Input: part model. Units: mm. Frame: model coordinates. Face numbers are marked on the shaded views. Coordinates: 2 decimals unless noted, no trailing zeros. Order: outer loops, then holes, each group sorted by start corner. A loop starts at its lowest first (then second) coordinate and runs counter-clockwise, first axis right, second up. Notation, with made-up numbers: (31.5, 41.25) -> (61.5, 41.25) arc R16 ccw to (61.5, 54.25) -> close; hole circle Ø4 at (0.25, 71.5). An arc over 180 degrees is marked (long way). Use one line per item in the form item = value. Start each with the question number.
1) Ray query, line 1 along X through (y, z) = (3, 0.5); line 2 along Z through (x, y) = (32.5, 0); line 3 along Y through (x, z) = (9, 0.25). Return the intervals inside material, ascending.
2) Pin query (flat end, axial travel): pin 1 (1 mm diameter, centred on x = 22.5, z = -0.5, fed in from +Y); pin 2 (0.7 mm diameter, centred on x = 2, y = 0.5, fed in from +Z); pin 3 (1 mm diameter, centred on x = 18.5, z = -2, fed in from +Y). Return the tip coordinate at first contact, or that it passes through.
3) Draft query along Y for the marked faces 1, 2 and 3. Return one class per face: pulls with the +Y half, pulls with the -Y half, needs draft (parallel to the pull), parting line crosses it, or undercut.
4) Section query A-A on x = 17. Output: boundary loops of the cut face in (y, z).
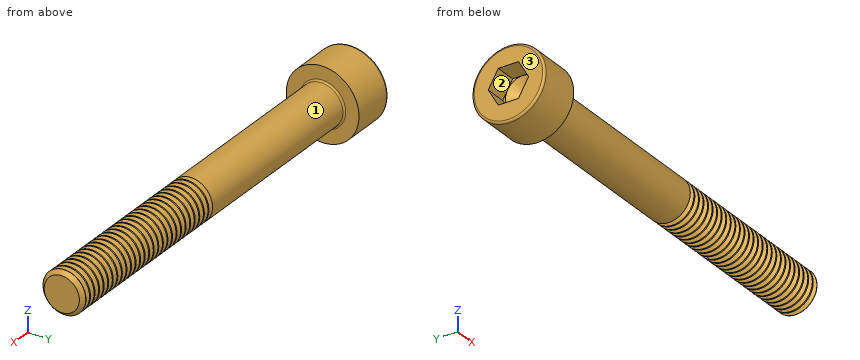
from build123d import *

# Parameters (mm, degrees)
FILLET1_R       = 0.2
FILLET2_R       = 0.25
HEX_2_DEPTH     = 2.5
THDSCHPAT_COUNT = 29
THDSCHPAT_PITCH = 0.785714286


with BuildPart() as part:
    # BodySke → Base-Revolve (revolve)
    with BuildSketch(Plane.XY):
        Polygon((0, 0), (0, 4.25), (5, 4.25), (5, 2.5), (49.555, 2.5), (50, 2.055), (50, 0), align=None)
    revolve(axis=Axis((-31.75, 0, 0), (1, 0, 0)))

    # Fillet1
    fillet1_edges = [part.edges().sort_by_distance(p)[0] for p in [
        (5, -2.5, 0),
    ]]
    fillet(fillet1_edges, radius=FILLET1_R)

    # Fillet2
    fillet2_edges = [part.edges().sort_by_distance(p)[0] for p in [
        (0, -4.25, 0),
    ]]
    fillet(fillet2_edges, radius=FILLET2_R)

    # Sketch2 → Hex-PreBroach (revolve, cut)
    with BuildSketch(Plane.XY):
        Polygon((0, 2.042), (2.5, 2.042), (3.67894925, 0), (0, 0), align=None)
    revolve(axis=Axis((0, 0, 0), (1, 0, 0)), mode=Mode.SUBTRACT)

    # Sketch3 → Hex 2 (cut)
    with BuildSketch(Plane(origin=(0, 0, 0), x_dir=(0, 0.5, 0.866025404), z_dir=(-1, 0, 0))):
        Polygon((1.17894925, 2.042), (-1.17894925, 2.042), (-2.357898499, 0), (-1.17894925, -2.042), (1.17894925, -2.042), (2.357898499, 0), align=None)
    extrude(amount=-HEX_2_DEPTH, mode=Mode.SUBTRACT)

    # ThdSchSke → ThreadSchematic (revolve, cut)
    with BuildSketch(Plane.XY):
        Polygon((28, -2.055), (27.688407645, -2.5), (27.688407645, -3.125), (28.311592355, -3.125), (28.311592355, -2.5), align=None)
    threadschematic = revolve(axis=Axis((-3.175, 0, 0), (1, 0, 0)), mode=Mode.SUBTRACT)

    # ThdSchPat: ThreadSchematic ×29
    with Locations(*[(i * THDSCHPAT_PITCH, 0, 0) for i in range(1, THDSCHPAT_COUNT)]):
        add(threadschematic, mode=Mode.SUBTRACT)


solid = part.part
Answers below:
q1.line_1 = 0 to 5
q1.line_2 = -2.36 to 2.36
q1.line_3 = -2.49 to 2.49
q2.pin_1 = 2.5
q2.pin_2 = 4.25
q2.pin_3 = 2
q3.face_1 = parting line crosses it
q3.face_2 = undercut
q3.face_3 = needs draft
q4.outline = circle Ø5 at (0, 0)
